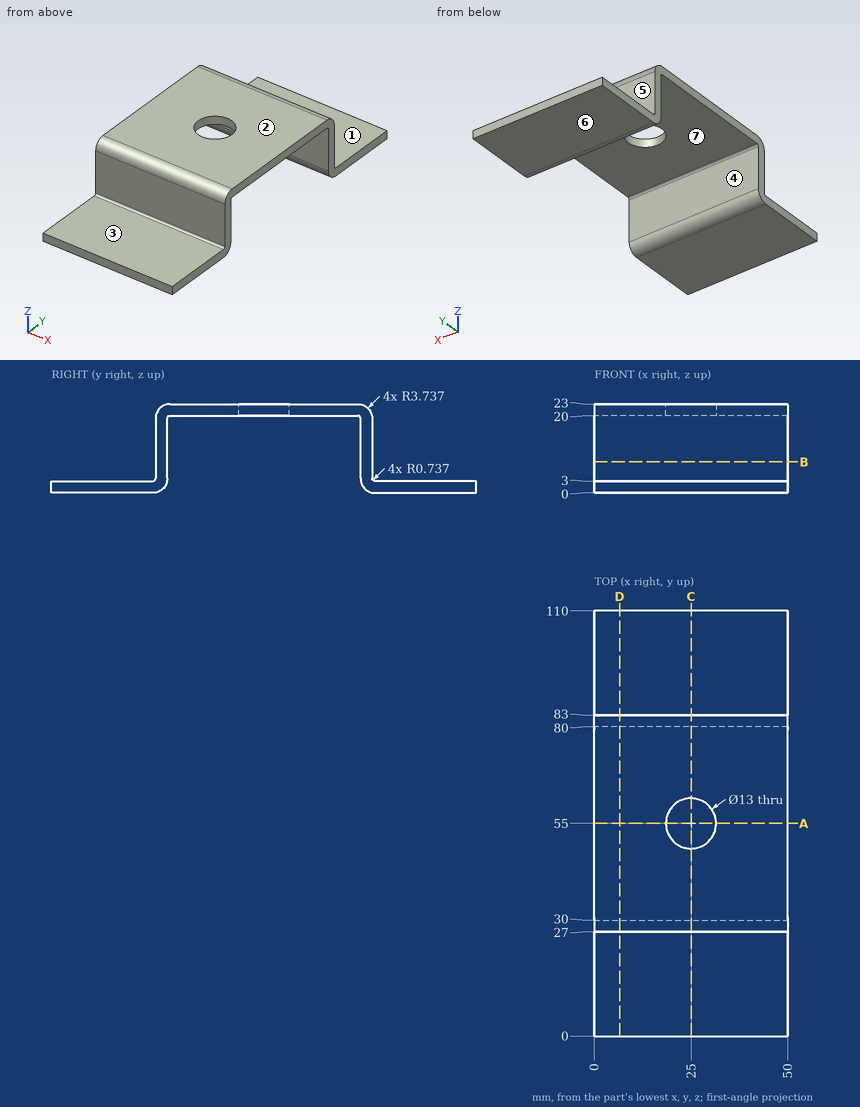
Geometry: see drawing. Coordinates: mm, zero at the bounding-box minimum. A direction names the side the tool comes from. Coordinates: 2 decimals unless noted, no trailing zeros. Loops run counter-clockwise (first coordinate to the right, second up) from the corner with the lowest first, then second, coordinate; pieces in that order, holes last.
Q1. Draft query along Y for the marked faces 5, 6 and 7. Return one class per face: +Y half, -Y half, draft (parallel to the pull), parting line (faces both ways), or undercut.
Q2. Cut plane B-B (z = 8). Output: boundary loops of the cut face in (x, y).
Q3. Set-up query: the marked faces 1, 2, 3 and 4. Return all of +Z, -Z, +X, -X, +Y, -Y with unobstructed straight access to the full face (end or side cutting, diameter ignored); none if empty.
Q4. Material intervals for line 1 (Y direction, x = 44, z = 13.25); line 2 (Z direction, x = 28.5, y = 40.5); line 3 (Y direction, x = 25, z = 20.8), sorted ascending.
Q5. Cut plane A-A (y = 55). Output: boundary loops of the cut face in (x, z).
Q6. Cut plane D-D (x = 6.5). Output: boundary loops of the cut face in (y, z).
Q7. Contact query for flat-ended pins moving along their axis: pin 1 (1 mm diameter, centred on x = 12, z = 2.5, fed in from -Y); pin 2 (8 mm diameter, centred on x = 14, z = 13.5, fed in from +Y); pin 3 (6 mm diameter, centred on x = 28, y = 38, fed in from -Z); pin 4 (13 mm diameter, centred on x = 29.5, y = 100, fed in from +Z). Output: stop coordinate, or through.
Q8. Cut plane C-C (x = 25). Output: boundary loops of the cut face in (y, z).
Working result:
1. face 5: +Y half
1. face 6: draft
1. face 7: undercut
2. outline: (0, 27) - (50, 27) - (50, 30) - (0, 30) - close; (0, 80) - (50, 80) - (50, 83) - (0, 83) - close
3. face 1: +Z, +X, -X, +Y
3. face 2: +Z, +X, -X, +Y, -Y
3. face 3: +Z, +X, -X, -Y
3. face 4: -Z, +X, -X
4. line 1: y = 27 to 30, 80 to 83
4. line 2: z = 20 to 23
4. line 3: y = 27.33 to 48.5, 61.5 to 82.67
5. outline: (0, 20) - (18.5, 20) - (18.5, 23) - (0, 23) - close; (31.5, 20) - (50, 20) - (50, 23) - (31.5, 23) - close
6. outline: (0, 0) - (26.26, 0) arc R3.74 ccw to (30, 3.74) - (30, 19.26) arc R0.74 cw to (30.74, 20) - (79.26, 20) arc R0.74 cw to (80, 19.26) - (80, 3.74) arc R3.74 ccw to (83.74, 0) - (110, 0) - (110, 3) - (83.74, 3) arc R0.74 cw to (83, 3.74) - (83, 19.26) arc R3.74 ccw to (79.26, 23) - (30.74, 23) arc R3.74 ccw to (27, 19.26) - (27, 3.74) arc R0.74 cw to (26.26, 3) - (0, 3) - close
7. pin 1: stops at y = 0
7. pin 2: stops at y = 83
7. pin 3: stops at z = 20
7. pin 4: stops at z = 3
8. outline: (0, 0) - (26.26, 0) arc R3.74 ccw to (30, 3.74) - (30, 19.26) arc R0.74 cw to (30.74, 20) - (48.5, 20) - (48.5, 23) - (30.74, 23) arc R3.74 ccw to (27, 19.26) - (27, 3.74) arc R0.74 cw to (26.26, 3) - (0, 3) - close; (61.5, 20) - (79.26, 20) arc R0.74 cw to (80, 19.26) - (80, 3.74) arc R3.74 ccw to (83.74, 0) - (110, 0) - (110, 3) - (83.74, 3) arc R0.74 cw to (83, 3.74) - (83, 19.26) arc R3.74 ccw to (79.26, 23) - (61.5, 23) - close
